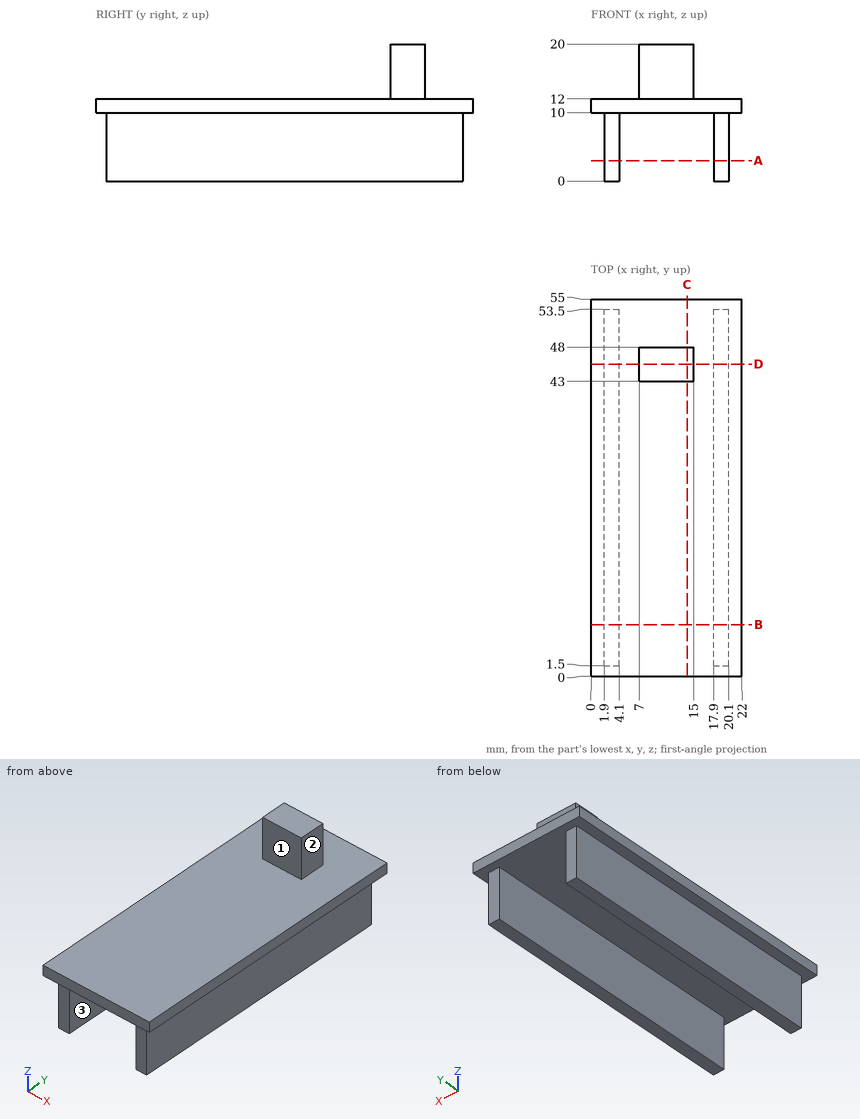
Could you check a few things on this drawing? It's one solid part, dimensions in mm from its lowest x, y, z. A direction names the side the tool comes from. Round coordinates to 2 decimals unless told otherwise and drop trailing zeros. Order: outer loops, then holes, each group sorted by start corner. A loop starts at its lowest first (then second) coordinate and runs counter-clockwise, first axis right, second up. Notation, with made-up numbers: M 79,88.5 L 133,88.5 A11 cw 133,105.5 Z; hole C 68,-15 d5. An arc over 180 degrees is marked long. One line per question, with ' | ' between items. Start each with the question number.
(1) For P1, Ø1.8, axis at x = 19, z = 4, coming from the +Y side; P2, Ø6, axis at x = 8, z = 5.5, coming from the -Y side; P3, Ø12, axis at x = 10.5, y = 23, coming from the -Z side; P4, Ø8, axis at y = 26.5, z = 5, coming from the +X side, each with a flat end and sliding along its axis, tell me the tip position at first contact or that it passes through.
(2) For the marked faces 1, 2 and 3, which set-ups out of +Z, -Z, +X, -X, +Y, -Y let a thin tool reach every point of the face, with its end or its side?
(3) Suppose I cut it at A-A on z = 3. List the corners of the cut face in (x, y) for me, then the cut area to 3 significant figures.
(4) Please list where these lines run through material, in increasing order: line 1 along X through (y, z) = (39, 6.5); line 2 along Z through (x, y) = (2.5, 49); line 3 along Z through (x, y) = (12, 13).
(5) Suppose I cut it at C-C on x = 14. List the corners of the cut face in (y, z) for me, then the cut area to 3 significant figures.
(6) Suppose I cut it at D-D on y = 45.5. List the corners of the cut face in (x, z) for me, then the cut area to 3 significant figures.
(7) Suppose I cut it at B-B on y = 7.5. List the corners of the cut face in (x, z) for me.
Geometry results:
1) P1: y = 53.5 | P2: through | P3: z = 10 | P4: x = 20.1
2) face 1: +Z, +X, -X, -Y | face 2: +Z, +X, +Y, -Y | face 3: -Z, +Y, -Y
3) outline: M 1.9,1.5 L 4.1,1.5 L 4.1,53.5 L 1.9,53.5 Z; M 17.9,1.5 L 20.1,1.5 L 20.1,53.5 L 17.9,53.5 Z | area: 229 mm²
4) line 1: 1.9 to 4.1, 17.9 to 20.1 | line 2: 0 to 12 | line 3: 10 to 12
5) outline: M 0,10 L 55,10 L 55,12 L 48,12 L 48,20 L 43,20 L 43,12 L 0,12 Z | area: 150 mm²
6) outline: M 0,10 L 1.9,10 L 1.9,0 L 4.1,0 L 4.1,10 L 17.9,10 L 17.9,0 L 20.1,0 L 20.1,10 L 22,10 L 22,12 L 15,12 L 15,20 L 7,20 L 7,12 L 0,12 Z | area: 152 mm²
7) outline: M 0,10 L 1.9,10 L 1.9,0 L 4.1,0 L 4.1,10 L 17.9,10 L 17.9,0 L 20.1,0 L 20.1,10 L 22,10 L 22,12 L 0,12 Z
